Geometry: final body of the model. Coordinates: model frame, mm. A direction names the side the tool comes from. Coordinates: 2 decimals unless noted, no trailing zeros. Write each loop counter-clockwise with the first axis right and the second up, starting at its lowest first coordinate (ties: lowest second). Pieces come first, ordered by that corner, then holes. Notation, with made-up numbers: (-35.5, 37) - (18.5, 37) arc R28 ccw to (18.5, 64) - close; hole circle Ø4 at (34.25, -33.5). An arc over 180 degrees is marked (long way). Answer as a JSON object with one key per item and string values. Group by question number.
Item 1: Section C-C on z = 1.55. Return loops of the section in (x, y).
Item 2: Line query: line 1 along X through (y, z) = (-58, 1.05); line 2 along Y through (x, z) = (-56, 1.2); line 3 along Y through (x, z) = (-45.5, 1.6). Output: solid intervals per line, ascending. Write a range as from..to.
Item 3: Mould query, pull axis Y, two halves, no side actions, for faces 1 (the cylindrical face through (-45.31, -67.23, 2.46)), 2 (the flat face through (-50, -69, 0)), 3 (the flat face through (-58.346, -84.175, 2.465)). Classes: pulls with the +Y half, pulls with the -Y half, needs draft (parallel to the pull), parting line crosses it, or undercut.
Item 4: Section D-D on y = -57.5. Return loops of the section in (x, z).
Item 5: Section A-A on x = -46. Return loops of the section in (y, z), and give its area (3 significant figures).
Item 6: Section B-B on y = -70. Return loops of the section in (x, z), and give its area (3 significant figures).
Item 7: Set-up query: faces 4 (the flat face through (-54.077, -64, 2)), 5 (the flat face through (-39.077, -74, 2)), 6 (the flat face through (-58.468, -89.175, 2.465)). Return all of +Z, -Z, +X, -X, +Y, -Y with unobstructed straight access to the full face (end or side cutting, diameter ignored); none if empty.
Item 8: First-contact query: pin 1 Ø1.5 at (y, z) = (-68, 3.5) entering from -X; pin 2 Ø1.5 at (y, z) = (-69, 3.5) entering from +X; pin 3 Ø1.5 at (x, y) = (-37, -69.5) entering from -Z. Flat tips, straight axial feed; report the tip coordinate or a pass-through.
```python
from build123d import *

# Parameters (mm, degrees)
F0_R     = 2.35
F1_DEPTH = 5


with BuildPart() as f1:
    # F0 (on Top) → F1 (new body)
    with BuildSketch(Plane.XY):
        Polygon((-39.076904, -51.710204), (-39.076904, -46.710204), (-54.076904, -46.710204), (-54.076904, -81.710204), (-54.076904, -86.710204), (-54.076904, -91.710204), (-39.076904, -91.710204), (-39.076904, -56.710204), align=None)
        with Locations((-46.576904, -69.210204)):
            Circle(F0_R, mode=Mode.SUBTRACT)
        Polygon((-30.41665, -51.710204), (-39.076904, -46.710204), (-39.076904, -51.710204), align=None)
        Polygon((-30.41665, -51.710204), (-39.076904, -51.710204), (-39.076904, -56.710204), align=None)
        Polygon((-54.076904, -86.710204), (-54.076904, -81.710204), (-62.737158, -86.710204), align=None)
        Polygon((-54.076904, -91.710204), (-54.076904, -86.710204), (-62.737158, -86.710204), align=None)
    extrude(amount=F1_DEPTH)


solid = f1.part
```
Checks:
{
 "1": {"outline": "(-62.74, -86.71) - (-54.08, -91.71) - (-39.08, -91.71) - (-39.08, -56.71) - (-30.42, -51.71) - (-39.08, -46.71) - (-54.08, -46.71) - (-54.08, -81.71) - close; hole circle Ø4.7 at (-46.58, -69.21)"},
 "2": {"line 1": "-54.08..-39.08", "line 2": "-90.6..-82.82", "line 3": "-91.71..-71.3, -67.12..-46.71"},
 "3": {"face 1": "undercut", "face 2": "needs draft", "face 3": "pulls with the +Y half"},
 "4": {"outline": "(-54.08, 0) - (-39.08, 0) - (-39.08, 5) - (-54.08, 5) - close"},
 "5": {"outline": "(-91.71, 0) - (-71.49, 0) - (-71.49, 5) - (-91.71, 5) - close; (-66.93, 0) - (-46.71, 0) - (-46.71, 5) - (-66.93, 5) - close", "area": "202 mm^2"},
 "6": {"outline": "(-54.08, 0) - (-48.79, 0) - (-48.79, 5) - (-54.08, 5) - close; (-44.36, 0) - (-39.08, 0) - (-39.08, 5) - (-44.36, 5) - close", "area": "52.9 mm^2"},
 "7": {"face 4": "+Z, -Z, -X, +Y", "face 5": "+Z, -Z, +X, -Y", "face 6": "+Z, -Z, -X, -Y"},
 "8": {"pin 1": "x = -54.08", "pin 2": "x = -39.08", "pin 3": "through"}
}
